The model under review builds one solid part; all positions refer to its coordinate system, in mm. Coordinates: 2 decimals unless noted, no trailing zeros. Order: outer loops, then holes, each group sorted by start corner. A loop starts at its lowest first (then second) coordinate and runs counter-clockwise, first axis right, second up. Notation, with made-up numbers: (79.25, 48) -> (99.25, 48) arc R16 ccw to (99.25, 70) -> close; hole circle Ø11 at (84, 36.5). An arc over 180 degrees is marked (long way). Use one line per item in the form item = value. Start each with the question number.
(1) Take a section at B-B (x = -16.5). State the section outline as (y, z) points.
(2) Take a section at C-C (z = 0.8). State the section outline as (x, y) points, then the cut area to 3 significant figures.
(3) Take a section at A-A (y = 15). State the section outline as (x, z) points.
(4) Wall thickness on line 1 along Y through (x, z) = (-10, 1); line 2 along X through (y, z) = (3, 0.15); line 3 along X through (y, z) = (21, 0.15): over which ranges is each line inside the solid? List them lowest first.
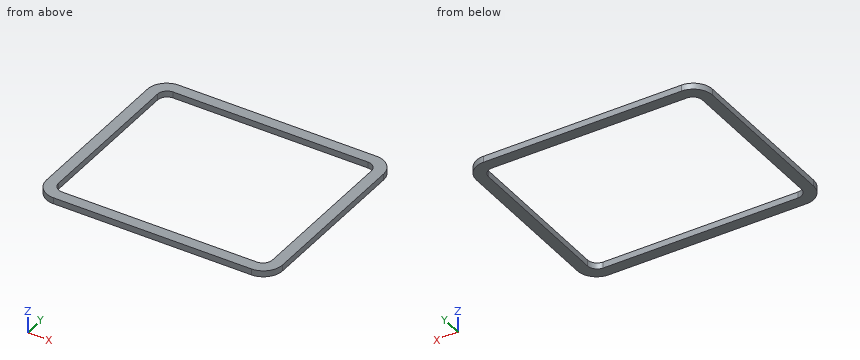
```python
from build123d import *

# Parameters (mm, degrees)
SKETCH2_W = 2.9
SKETCH2_H = 1.6
FILLET1_R = 5
FILLET2_R = 2.5


with BuildPart() as part:
    # Sweep1: sweep along a path in Sketch1
    with BuildLine(Plane.XY) as sweep1_path:
        Line((-30.7, 25.75), (30.7, 25.75))
        Line((30.7, 25.75), (30.7, -25.75))
        Line((30.7, -25.75), (-30.7, -25.75))
        Line((-30.7, -25.75), (-30.7, 25.75))
    # Sketch2 → Sweep1 (sweep)
    with BuildSketch(Plane(origin=(0, 0, 0), x_dir=(1, 0, 0), z_dir=(0, 1, 0))):
        with Locations((-29.25, -0.8)):
            Rectangle(SKETCH2_W, SKETCH2_H)
    sweep(path=sweep1_path.line, transition=Transition.RIGHT)

    # Fillet1
    fillet1_edges = [part.edges().sort_by_distance(p)[0] for p in [
        (30.7, -25.75, 0.8),
        (-30.7, -25.75, 0.8),
        (30.7, 25.75, 0.8),
        (-30.7, 25.75, 0.8),
    ]]
    fillet(fillet1_edges, radius=FILLET1_R)

    # Fillet2
    fillet2_edges = [part.edges().sort_by_distance(p)[0] for p in [
        (27.8, -22.85, 0.8),
        (-27.8, -22.85, 0.8),
        (27.8, 22.85, 0.8),
        (-27.8, 22.85, 0.8),
    ]]
    fillet(fillet2_edges, radius=FILLET2_R)


solid = part.part
```
Findings:
q1.outline = (-25.75, 0) -> (-22.85, 0) -> (-22.85, 1.6) -> (-25.75, 1.6) -> close; (22.85, 0) -> (25.75, 0) -> (25.75, 1.6) -> (22.85, 1.6) -> close
q2.outline = (-30.7, -20.75) arc R5 ccw to (-25.7, -25.75) -> (25.7, -25.75) arc R5 ccw to (30.7, -20.75) -> (30.7, 20.75) arc R5 ccw to (25.7, 25.75) -> (-25.7, 25.75) arc R5 ccw to (-30.7, 20.75) -> close; hole (-27.8, -20.35) arc R2.5 ccw to (-25.3, -22.85) -> (25.3, -22.85) arc R2.5 ccw to (27.8, -20.35) -> (27.8, 20.35) arc R2.5 ccw to (25.3, 22.85) -> (-25.3, 22.85) arc R2.5 ccw to (-27.8, 20.35) -> close
q2.area = 605 mm²
q3.outline = (-30.7, 0) -> (-27.8, 0) -> (-27.8, 1.6) -> (-30.7, 1.6) -> close; (27.8, 0) -> (30.7, 0) -> (30.7, 1.6) -> (27.8, 1.6) -> close
q4.line_1 = -25.75 to -22.85, 22.85 to 25.75
q4.line_2 = -30.7 to -27.8, 27.8 to 30.7
q4.line_3 = -30.69 to -27.71, 27.71 to 30.69
